Autodesk Inventor part; units mm, degrees
ref_plane "YZ Plane" through (0, 0, 0) normal (1, 0, 0) x (0, 1, 0)
ref_plane "XZ Plane" through (0, 0, 0) normal (0, 1, 0) x (-1, 0, 0)
ref_plane "XY Plane" through (0, 0, 0) normal (0, 0, 1) x (1, 0, 0)
sketch "スケッチ1" plane through (0, 0, 0) normal (0, 0, 1) x (1, 0, 0)
  line L0 (52.125, -16.25) -> (-52.125, -16.25)
  line L1 (-52.125, -16.25) -> (-52.125, 16.25)
  line L2 (-52.125, 16.25) -> (52.125, 16.25)
  line L3 (52.125, 16.25) -> (52.125, -16.25)
  line L4 (52.125, -16.25) -> (-52.125, 16.25) construction
  line L5 (-52.125, -16.25) -> (52.125, 16.25) construction
  point P0 (0, 0)
  dimension "d0" = 104.25
  dimension "d1" = 32.5
extrude "枠" add sketch "スケッチ1" along normal blind 19
sketch "スケッチ2" plane through (0, 0, 0) normal (0, 0, -1) x (-1, 0, 0)
  line L0 (50.125, -14.25) -> (-50.125, -14.25)
  line L1 (-50.125, -14.25) -> (-50.125, 14.25)
  line L2 (-50.125, 14.25) -> (50.125, 14.25)
  line L3 (50.125, 14.25) -> (50.125, -14.25)
  line L4 (50.125, -14.25) -> (-50.125, 14.25) construction
  line L5 (-50.125, -14.25) -> (50.125, 14.25) construction
  point P0 (0, 0)
  dimension "d4" = 100.25
  dimension "d5" = 28.5
extrude "本体" cut sketch "スケッチ2" against normal blind 12
sketch "スケッチ3" plane through (-52.125, -16.25, 0) normal (-1, 0, 0) x (0, 0, 1)
  line L0 (2, 2) -> (14, 2)
  line L1 (14, 2) -> (14, 30.5)
  line L2 (14, 30.5) -> (2, 30.5)
  line L3 (2, 30.5) -> (2, 2)
  line L4 (19, 32.5) -> (19, 0)
  line L5 (0, 0) -> (19, 0)
  line L6 (0, 0) -> (0, 32.5)
  line L7 (0, 32.5) -> (19, 32.5)
  point P0 (0, 16.25)
  dimension "d8" = 5
  dimension "d9" = 28.5
  dimension "d10" = 2
  dimension "d11" = 12
  dimension "d12" = 2
  dimension "d13" = 2
extrude "入口" cut sketch "スケッチ3" against normal blind 102.25 contours L3 L2 L1 L0
sketch "スケッチ4" plane through (-52.125, -16.25, 0) normal (0, -1, 0) x (1, 0, 0)
  line L0 (98.25, 2) -> (14, 2)
  line L1 (14, 2) -> (14, 14)
  line L2 (14, 14) -> (98.25, 14)
  line L3 (98.25, 14) -> (98.25, 2)
  line L4 (104.25, 0) -> (104.25, 19)
  line L5 (0, 0) -> (0, 19)
  line L6 (0, 19) -> (104.25, 19)
  line L7 (104.25, 0) -> (0, 0)
  point P0 (52.125, 0)
  dimension "d16" = 6
  dimension "d17" = 14
  dimension "d18" = 5
  dimension "d19" = 2
extrude "USB穴" cut sketch "スケッチ4" against normal blind 2 contours L0 L1 L2 L3
sketch "スケッチ6" plane through (-52.125, -16.25, 0) normal (-1, 0, 0) x (0, 0, 1)
  line L0 (14, 30.5) -> (14, 2)
  line L1 (14, 4) -> (17, 4)
  line L2 (17, 4) -> (17, 13)
  line L3 (17, 13) -> (14, 13)
  line L4 (14, 13) -> (14, 4)
  line L5 (14, 17) -> (17, 17)
  line L6 (17, 17) -> (17, 26)
  line L7 (17, 26) -> (14, 26)
  line L8 (14, 26) -> (14, 17)
  line L9 (14, 2) -> (2, 2)
  point P0 (0, 16.25)
  dimension "d22" = 9
  dimension "d23" = 9
  dimension "d24" = 3
  dimension "d25" = 2
  dimension "d26" = 4
extrude "ネジ溝" cut sketch "スケッチ6" against normal blind 102.25
sketch "スケッチ7" plane through (-52.125, -12.25, 17) normal (0, 0, -1) x (-1, 0, 0)
  line L0 (-88.25, 5.2069) -> (-24.75, 5.2069)
  line L1 (-24.75, 5.2069) -> (-24.75, 18.2069)
  line L2 (-24.75, 18.2069) -> (-88.25, 18.2069)
  line L3 (-88.25, 18.2069) -> (-88.25, 5.2069)
  line L4 (-104.25, 28.5) -> (-104.25, -4)
  point P0 (-52.125, 12.25)
  dimension "d29" = 13
  dimension "d30" = 63.5
  dimension "d31" = 16
hole "穴1" at (36.125, -7.0431, 17) at (-27.375, -7.0431, 17) at (-27.375, 5.9569, 17) at (36.125, 5.9569, 17) direction (0, 0, 1) diameter 3 depth 8 tip angle 118
sketch "スケッチ10" plane through (0, 0, 0) normal (0, 0, -1) x (-1, 0, 0)
  line L0 (52.125, -16.25) -> (-52.125, -16.25)
  line L1 (-52.125, -16.25) -> (52.125, -16.25)
  line L2 (52.125, -14.25) -> (38.125, -14.25)
  line L3 (52.125, 16.25) -> (52.125, -16.25)
  line L4 (52.125, -16.25) -> (52.125, 16.25)
  line L5 (-52.125, 16.25) -> (52.125, 16.25)
  line L6 (52.125, 16.25) -> (-52.125, 16.25)
  line L7 (-52.125, -16.25) -> (-52.125, 16.25)
  line L8 (-52.125, 16.25) -> (-52.125, -16.25)
  line L9 (-48.125, -12.25) -> (48.125, -12.25)
  line L10 (50.125, -14.25) -> (-50.125, -14.25)
  line L11 (48.125, -12.25) -> (48.125, 12.25)
  line L12 (48.125, 12.25) -> (-48.125, 12.25)
  line L13 (-48.125, 12.25) -> (-48.125, -12.25)
  point P0 (0, 0)
  dimension "d40" = 4
  dimension "d41" = 4
  dimension "d42" = 4
  dimension "d43" = 4
extrude "蓋" add sketch "スケッチ10" along normal blind 1
sketch "スケッチ13" plane through (-52.125, -16.25, 19) normal (-1, 0, 0) x (0, 0, 1)
  line L0 (0, 0) -> (-20, 0)
  line L1 (0, 32.5) -> (0, 0)
  line L2 (-20, 0) -> (0, 0)
  line L3 (0, 0) -> (0, 32.5)
  line L4 (0, 32.5) -> (-20, 32.5)
  line L5 (-20, 32.5) -> (-20, 0)
  point P0 (-19, 16.25)
extrude "調整" cut sketch "スケッチ13" against normal blind 2
properties part number "usbhub_holder_new"
The model under review builds one solid part; all positions refer to its coordinate system, in mm. A direction names the side the tool comes from. Round coordinates to 2 decimals unless told otherwise and drop trailing zeros. Write each loop counter-clockwise with the first axis right and the second up, starting at its lowest first coordinate (ties: lowest second). Pieces come first, ordered by that corner, then holes. Notation, with made-up numbers: M -40,-36 L 5,-36 A22 ccw 5,-3 Z; hole C 87,57 d7. An arc over 180 degrees is marked long. Use a Markdown table: item, result. Add a question column.
Q1. To check wall thickness, follow line 1 (Y direction, x = -40.5, z = 16); line 2 (Y direction, x = -1, z = 0.25); line 3 (Z direction, x = -20, y = 7.5). State the ranges of each line that lie inside material, in increasing order.
Q2. We need section D-D, the plane y = -7.5. State the section outline as (x, z) points (3 decimals).
Q3. We need section B-B, the plane x = 12. State the section outline as (y, z) points, plus the area to 4 significant figures.
Q4. Machinability: for faces 4 (the face through (5, -15, 2)), 5 (the face through (-28.862, -7.238, 18.014)), 6 (the face through (-7.7, -14.25, 1.8)), which of the approach directions +Z, -Z, +X, -X, +Y, -Y give a long, thin tool a straight path to every point of the face, cutting with its end or side? Answer none if there is none.
Q5. Insertion check: pin 1 (1 mm diameter, centred on y = 4.5, z = 1, fed in from -X) (3 decimals); pin 2 (7 mm diameter, centred on x = -7, y = 3.5, fed in from -Z); pin 3 (5 mm diameter, centred on x = 36.12, y = 5.96, fed in from -Z). Each pin has a flat end and moves straight along its axis. Give the tip position at first contact, or say it passes through.
Q6. The part is to be moulded in two halves that separate along X. For faces 1 (the face through (2, 16.25, 9)), 2 (the face through (46.125, -15, 8)), 3 (the face through (52.125, 0, 9)), say which applies: pulls with the +X half, pulls with the -X half, needs draft (parallel to the pull), parting line crosses it, or undercut.
Q7. We need section A-A, the plane z = 7.5. State the section outline as (x, y) points (3 decimals), plus the area to 4 significant figures.
Q8. We need section C-C, the plane y = 2.5. State the section outline as (x, z) points (3 decimals), plus the area to 4 significant figures.
Findings below:
| question | item | result |
|---|---|---|
| 1 | line 1 | y = -16.25 to -12.25, -3.25 to 0.75, 9.75 to 16.25 |
| 1 | line 2 | y = -16.25 to -14.25, 14.25 to 16.25 |
| 1 | line 3 | z = 17 to 19 |
| 2 | outline | M -50.125,-1 L -48.125,-1 L -48.125,0 L -50.125,0 Z; M -50.125,17 L -28.804,17 L -28.804,19 L -50.125,19 Z; M -25.946,17 L 34.696,17 L 34.696,19 L -25.946,19 Z; M 37.554,17 L 50.125,17 L 50.125,0 L 48.125,0 L 48.125,-1 L 52.125,-1 L 52.125,19 L 37.554,19 Z |
| 3 | outline | M -16.25,-1 L -12.25,-1 L -12.25,0 L -14.25,0 L -14.25,2 L -16.25,2 Z; M -16.25,14 L -12.25,14 L -12.25,17 L -3.25,17 L -3.25,14 L 0.75,14 L 0.75,17 L 9.75,17 L 9.75,14 L 14.25,14 L 14.25,0 L 12.25,0 L 12.25,-1 L 16.25,-1 L 16.25,19 L -16.25,19 Z |
| 3 | area | 148.5 mm² |
| 4 | face 4 | -Y |
| 4 | face 5 | +Z, -Z |
| 4 | face 6 | -X |
| 5 | pin 1 | stops at x = 50.125 |
| 5 | pin 2 | stops at z = 14 |
| 5 | pin 3 | stops at z = 17 |
| 6 | face 1 | needs draft |
| 6 | face 2 | undercut |
| 6 | face 3 | pulls with the +X half |
| 7 | outline | M -50.125,-16.25 L -38.125,-16.25 L -38.125,-14.25 L -50.125,-14.25 Z; M -50.125,14.25 L 50.125,14.25 L 50.125,-14.25 L 46.125,-14.25 L 46.125,-16.25 L 52.125,-16.25 L 52.125,16.25 L -50.125,16.25 Z |
| 7 | area | 297.5 mm² |
| 8 | outline | M -50.125,-1 L -48.125,-1 L -48.125,0 L -50.125,0 Z; M -50.125,17 L 50.125,17 L 50.125,0 L 48.125,0 L 48.125,-1 L 52.125,-1 L 52.125,19 L -50.125,19 Z |
| 8 | area | 244.5 mm² |
